Design review of the part built by this model. Coordinates are the model's own, in mm. Give positions to 0.01 mm unless a question says otherwise; leave off trailing zeros. Loops run counter-clockwise (first coordinate to the right, second up) from the corner with the lowest first, then second, coordinate; pieces in that order, holes last. Notation, with made-up numbers: (-16, 80.5) - (31, 80.5) arc R34 cw to (31, 115.5) - close; hole circle Ø1 at (63.25, -32). An arc over 180 degrees is marked (long way). Write each question's results on one line, items separated by ' | '.
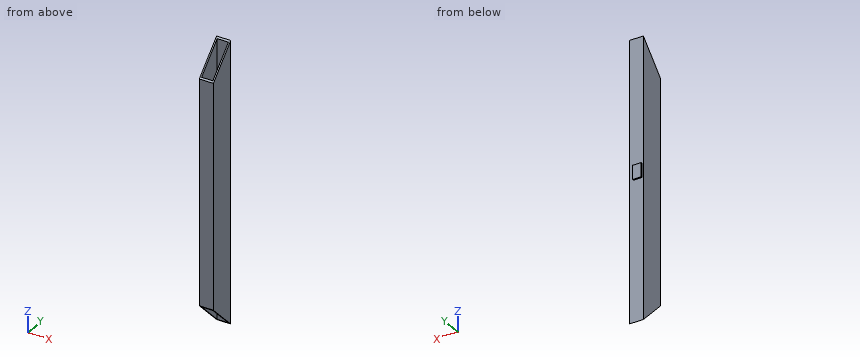
Autodesk Inventor part; units mm, degrees
ref_plane "YZ Plane" through (0, 0, 0) normal (1, 0, 0) x (0, 1, 0)
ref_plane "XZ Plane" through (0, 0, 0) normal (0, 1, 0) x (-1, 0, 0)
ref_plane "XY Plane" through (0, 0, 0) normal (0, 0, 1) x (1, 0, 0)
sketch "Sketch2" plane through (0, 0, 0) normal (0, 0, 1) x (1, 0, 0)
  line L0 (-9.4777, 15.0257) -> (40.5223, 15.0257)
  line L1 (40.5223, 15.0257) -> (40.5223, -84.9743)
  line L2 (40.5223, -84.9743) -> (-9.4777, -84.9743)
  line L3 (-9.4777, -84.9743) -> (-9.4777, 15.0257)
  line L4 (35.5223, 10.0257) -> (-4.4777, 10.0257)
  line L5 (-4.4777, 10.0257) -> (-4.4777, -79.9743)
  line L6 (-4.4777, -79.9743) -> (35.5223, -79.9743)
  line L7 (35.5223, -79.9743) -> (35.5223, 10.0257)
  point P0 (0, 0)
  point P1 (0, 0)
  dimension "d6" = 50
  dimension "d7" = 100
  dimension "d8" = 5
  dimension "d9" = 90
  dimension "d10" = 5
  dimension "d11" = 40
extrude "Extrusion1" add sketch "Sketch2" along normal blind 1000
sketch "Sketch3" plane through (40.5223, -84.9743, 0) normal (1, 0, 0) x (0, 0, -1)
  line L0 (0, 100) -> (-100, 0)
  line L1 (0, 100) -> (141.4214, 100) construction
  line L2 (0, 0) -> (0, 100)
  line L3 (0, 100) -> (0, 0)
  line L4 (0, 0) -> (-100, 0)
  line L5 (0, 0) -> (-1000, 0)
  line L6 (0, 100) -> (-1000, 100)
  line L7 (-1000, 100) -> (-900, 0)
  line L8 (-1000, 100) -> (-858.5786, 100) construction
  line L9 (-1000, 100) -> (-1000, 0)
  line L10 (-1000, 0) -> (-900, 0)
  point P0 (0, 84.9743)
  dimension "d14" = 135
  dimension "d15" = 45
extrude "Extrusion2" cut sketch "Sketch3" against normal blind 1000 contours L2 L4 L0 | L7 L5 L9
sketch "Sketch5" plane through (-9.4777, 15.0257, 0) normal (0, 1, 0) x (1, 0, 0)
  line L0 (5, -552.5) -> (35.1644, -552.5)
  line L1 (35.1644, -552.5) -> (35.1644, -502.5)
  line L2 (35.1644, -502.5) -> (5, -502.5)
  line L3 (5, -502.5) -> (5, -552.5)
  line L4 (0, 0) -> (0, -1000)
  line L5 (50, 0) -> (0, 0)
  point P0 (9.4777, 0)
  dimension "d23" = 5
  dimension "d24" = 50
  dimension "d25" = 502.5
extrude "Extrusion4" add sketch "Sketch5" along normal blind 5
properties part number "PerfilH1"
(1) Take a section at B-B on z = 378. Give the boundary of the cut face in (x, y), plus the area to 3 significant figures.
Answers below:
outline: (-9.48, -84.97) - (40.52, -84.97) - (40.52, 15.03) - (-9.48, 15.03) - close; hole (-4.48, -79.97) - (35.52, -79.97) - (35.52, 10.03) - (-4.48, 10.03) - close | area: 1,400 mm2
(2) Wall thickness on line 1 along Y through (x, z) = (4, 546.5); line 2 along X through (y, z) = (0, 629); line 3 along Y through (x, z) = (11, 184): over which ranges is each line inside the solid? List them lowest first. Write a range as from..to.
Answers below:
line 1: -84.97..-79.97, 10.03..20.03 | line 2: -9.48..-4.48, 35.52..40.52 | line 3: -84.97..-79.97, 10.03..15.03
(3) Take a section at C-C on y = -5. Give the boundary of the cut face in (x, z), plus the area to 3 significant figures.
Answers below:
outline: (-9.48, 20.03) - (-4.48, 20.03) - (-4.48, 979.97) - (-9.48, 979.97) - close; (35.52, 20.03) - (40.52, 20.03) - (40.52, 979.97) - (35.52, 979.97) - close | area: 9,600 mm2
(4) Take a section at A-A on x = 12.5. Give the boundary of the cut face in (y, z).
Answers below:
outline: (-84.97, 100) - (-79.97, 95) - (-79.97, 905) - (-84.97, 900) - close; (10.03, 5) - (15.03, 0) - (15.03, 502.5) - (20.03, 502.5) - (20.03, 552.5) - (15.03, 552.5) - (15.03, 1000) - (10.03, 995) - close
(5) Insertion check: P1, Ø1.5, axis at x = 15.5, z = 679.5, coming from the +Y side; P2, Ø1.5, axis at y = 18, z = 539.5, coming from the -X side; P3, Ø12, axis at x = 31, y = -38.5, coming from the +Z side; P4, Ø3, axis at x = 26, y = 7.5, coming from the -Z side. Each pin has a flat end and moves straight along its axis. Give the tip position at first contact, or say it passes through.
Answers below:
P1: y = 15.03 | P2: x = -4.48 | P3: z = 950.42 | P4: through
(6) Take a section at D-D on y = -56. Give the boundary of the cut face in (x, z), plus the area to 3 significant figures.
Answers below:
outline: (-9.48, 71.03) - (-4.48, 71.03) - (-4.48, 928.97) - (-9.48, 928.97) - close; (35.52, 71.03) - (40.52, 71.03) - (40.52, 928.97) - (35.52, 928.97) - close | area: 8,580 mm2
